Check sheet for the modelled part. Datum: model origin and axes. Units: mm. Face numbers are marked on the shaded views. Coordinates: 2 decimals unless noted, no trailing zeros. Write each loop counter-clockwise with the first axis right and the second up, starting at its lowest first coordinate (ties: lowest second). Pieces come first, ordered by that corner, then holes. Notation, with made-up numbers: (-39.5, 43.5) - (-34.5, 43.5) arc R27 cw to (-34.5, 77.5) - close; hole circle Ø7 at (85.5, -13.75). An arc over 180 degrees is marked (long way). Use one line per item in the form item = value. Start each with the question number.
1. Scan line: line 1 along Z through (x, y) = (19, -33.5). Record every from-to range of solid material in increasing order.
2. Draft check along X on the marked faces 1, 2 and 3. Enter one of: +X half, -X half, draft (parallel to the pull), parting line (faces both ways), or undercut.
3. Cross-section at A-A on y = -60.5. Record the boundary of the cut face in (x, z).
4. Go/stop test with a flat-tipped pin: pin 1 Ø3 at (x, y) = (-32.5, -18) entering from +Z. Record where the tip stops, or that it passes through.
5. Cross-section at B-B on x = 27.5. Record the boundary of the cut face in (y, z), then the cut area to 3 significant figures.
```python
from build123d import *

# Parameters (mm, degrees)
SKETCH1_W           = 370
SKETCH1_H           = 315
BOSS_EXTRUDE1_DEPTH = 250
FILLET2_R           = 5
SKETCH3_W           = 350
SKETCH3_H           = 280
CUT_EXTRUDE1_DEPTH  = 5
FILLET3_R           = 2
SCALE3_SCALE        = 0.3


with BuildPart() as part:
    # Sketch1 → Boss-Extrude1 (new body)
    with BuildSketch(Plane.XY):
        with Locations((7.880798198, -42.761829759)):
            Rectangle(SKETCH1_W, SKETCH1_H)
    extrude(amount=BOSS_EXTRUDE1_DEPTH)

    # Fillet2
    fillet2_edges = [part.edges().sort_by_distance(p)[0] for p in [
        (-177.119201802, 114.738170241, 125),
        (192.880798198, 114.738170241, 125),
        (192.880798198, -200.261829759, 125),
        (-177.119201802, -200.261829759, 125),
    ]]
    fillet(fillet2_edges, radius=FILLET2_R)

    # Sketch3 → Cut-Extrude1 (cut)
    with BuildSketch(Plane.XY.offset(250)):
        with Locations((7.880798198, -35.261829759)):
            Rectangle(SKETCH3_W, SKETCH3_H)
    extrude(amount=-CUT_EXTRUDE1_DEPTH, mode=Mode.SUBTRACT)

    # Fillet3
    fillet3_edges = [part.edges().sort_by_distance(p)[0] for p in [
        (-167.119201802, -175.261829759, 247.5),
        (-167.119201802, 104.738170241, 247.5),
        (182.880798198, 104.738170241, 247.5),
        (182.880798198, -175.261829759, 247.5),
    ]]
    fillet(fillet3_edges, radius=FILLET3_R)


with BuildPart() as part_1:
    # Scale3: scaled about (7.880798198, -42.890132661, 122.904385933)
    add(part.part.scale(SCALE3_SCALE).moved(Location((5.516558739, -30.023092863, 86.033070153))))


solid = part_1.part
```
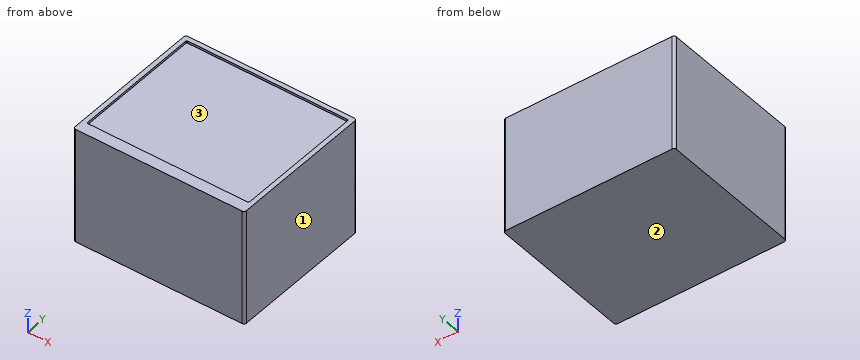
Final values:
q1.line_1 = 86.03 to 159.53
q2.face_1 = +X half
q2.face_2 = draft
q2.face_3 = undercut
q3.outline = (-47.62, 86.03) - (63.38, 86.03) - (63.38, 161.03) - (60.38, 161.03) - (60.38, 159.53) - (-44.62, 159.53) - (-44.62, 161.03) - (-47.62, 161.03) - close
q4.pin_1 = 159.53
q5.outline = (-90.1, 86.03) - (4.4, 86.03) - (4.4, 161.03) - (1.4, 161.03) - (1.4, 159.53) - (-82.6, 159.53) - (-82.6, 161.03) - (-90.1, 161.03) - close
q5.area = 6,960 mm²
